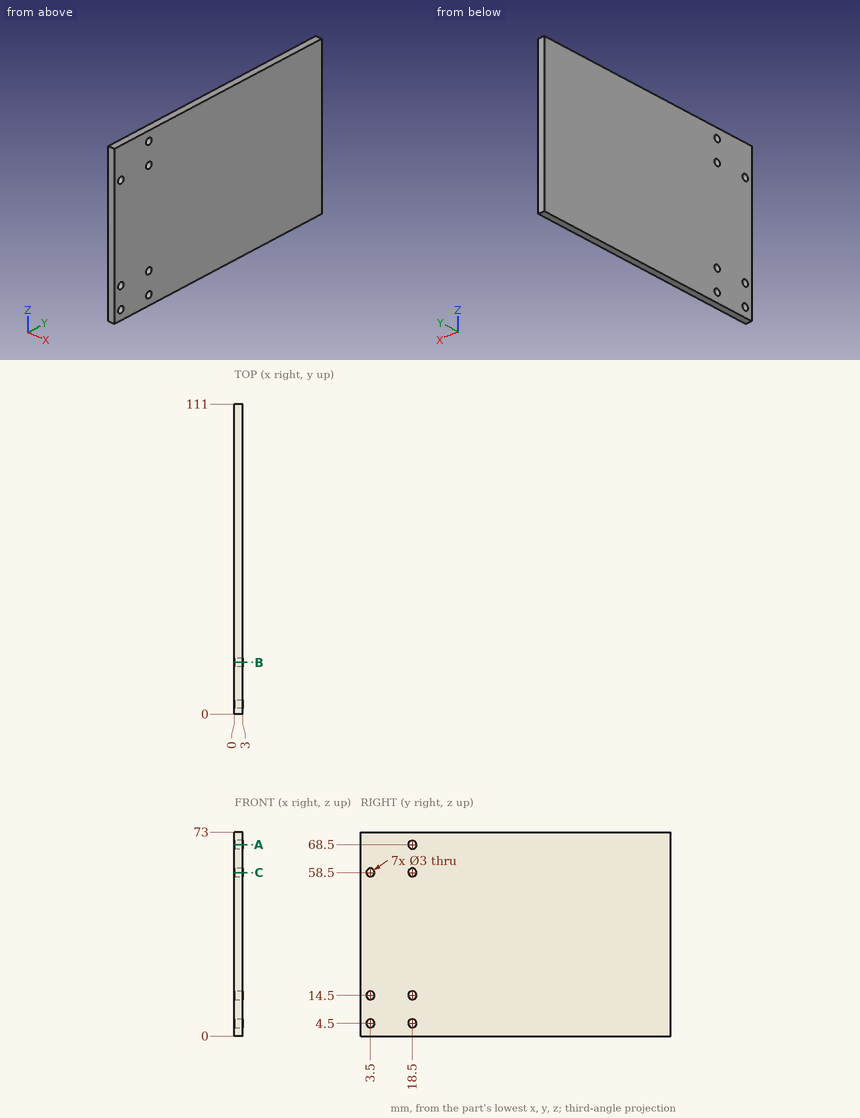
Job drawing, mm, ordinate dimensions from the low corner. One solid piece. Give positions to 0.01 mm unless a question says otherwise; leave off trailing zeros. Order: outer loops, then holes, each group sorted by start corner. A loop starts at its lowest first (then second) coordinate and runs counter-clockwise, first axis right, second up. Notation, with made-up numbers: M -27.75,45.25 L -23.75,45.25 A18 ccw -23.75,60.25 Z; hole C 14,23.5 d11. An arc over 180 degrees is marked long. Put each result on its own line as item: value. Start each with the question number.
(1) Band-saw the part on C-C on z = 58.5. Give the cut face in (x, y).
(2) Band-saw the part on B-B on y = 18.5. Give the cut face in (x, z), then the cut area to 3 significant figures.
(3) Band-saw the part on A-A on z = 68.5. Give the cut face in (x, y).
(4) Drill centre lines: L1, parallel to Y at x = 1.45, z = 4.5; L2, parallel to Y at x = 2.35, z = 68.5; L3, parallel to Y at x = 0.65, z = 67.5. Where is each one in solid material? Low to high. Write a range as [from, to].
(5) Pin check, flat tips, straight feed: pin 1 Ø2.5 at (y, z) = (3.5, 58.5) entering from -X; pin 2 Ø1.5 at (x, z) = (2.5, 20.5) entering from -Y. Stop position of each tip, or through.
Results below:
1. outline: M 0,0 L 3,0 L 3,2 L 0,2 Z; M 0,5 L 3,5 L 3,17 L 0,17 Z; M 0,20 L 3,20 L 3,111 L 0,111 Z
2. outline: M 0,0 L 3,0 L 3,3 L 0,3 Z; M 0,6 L 3,6 L 3,13 L 0,13 Z; M 0,16 L 3,16 L 3,57 L 0,57 Z; M 0,60 L 3,60 L 3,67 L 0,67 Z; M 0,70 L 3,70 L 3,73 L 0,73 Z
2. area: 183 mm2
3. outline: M 0,0 L 3,0 L 3,17 L 0,17 Z; M 0,20 L 3,20 L 3,111 L 0,111 Z
4. L1: y = [0, 2], [5, 17], [20, 111]
4. L2: y = [0, 17], [20, 111]
4. L3: y = [0, 17.38], [19.62, 111]
5. pin 1: passes through
5. pin 2: stops at y = 0
